Work out the finished part from the listing and answer in its coordinate system (mm). Face numbers are marked on the shaded views. Coordinates: 2 decimals unless noted, no trailing zeros. Loops run counter-clockwise (first coordinate to the right, second up) from the corner with the lowest first, then second, coordinate; pieces in that order, holes last. Notation, with made-up numbers: (88, 4) -> (113, 4) arc R14 cw to (113, 21) -> close; hole circle Ø6 at (66.25, -0.5). An arc over 180 degrees is marked (long way). Answer as CSV lines item,"result".
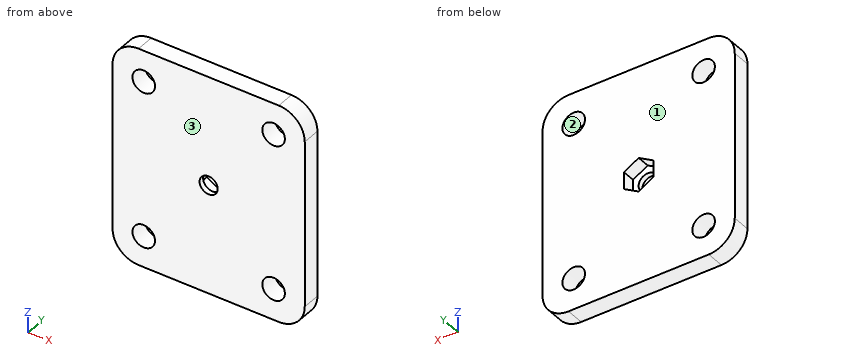
Autodesk Inventor part; units mm, degrees
ref_plane "YZ Plane" through (0, 0, 0) normal (1, 0, 0) x (0, 1, 0)
ref_plane "XZ Plane" through (0, 0, 0) normal (0, 1, 0) x (-1, 0, 0)
ref_plane "XY Plane" through (0, 0, 0) normal (0, 0, 1) x (1, 0, 0)
sketch "Sketch1" plane through (0, 0, 0) normal (0, 1, 0) x (-1, 0, 0)
  line L0 (37, 42) -> (-37, 42)
  line L1 (-37, 42) -> (-37, -42)
  line L2 (-37, -42) -> (37, -42)
  line L3 (37, -42) -> (37, 42)
  line L4 (37, 42) -> (-37, -42) construction
  line L5 (-37, 42) -> (37, -42) construction
  circle A0 centre (25, 30) radius 4.35
  circle A1 centre (25, -30) radius 4.35
  circle A2 centre (-25, 30) radius 4.35
  circle A3 centre (-25, -30) radius 4.35
  point P0 (0, 0)
  dimension "d0" = 74
  dimension "d1" = 84
  dimension "d4" = 60
  dimension "d7" = 50
  dimension "d10" = 8.7
  dimension "d11" = 12
  dimension "d12" = 12
extrude "Extrusion1" add sketch "Sketch1" along normal blind 7
fillet "Fillet1" radius 10 4 edges at (-37, 3.5, 42) (37, 3.5, 42) (37, 3.5, -42) (-37, 3.5, -42)
sketch "Sketch2" plane through (0, 7, 0) normal (0, 1, 0) x (1, 0, 0)
  line L0 (0, 6.5241) -> (5.65, 3.262)
  line L1 (5.65, 3.262) -> (5.65, -3.262)
  line L2 (5.65, -3.262) -> (0, -6.5241)
  line L3 (0, -6.5241) -> (-5.65, -3.262)
  line L4 (-5.65, -3.262) -> (-5.65, 3.262)
  line L5 (-5.65, 3.262) -> (0, 6.5241)
  point P0 (0, 0)
  point P1 (0, 0)
  dimension "d16" = 11.3
extrude "Extrusion2" cut sketch "Sketch2" against normal blind 5
sketch "Sketch3" plane through (0, 2, 0) normal (0, 1, 0) x (1, 0, 0)
  circle A0 centre (0, 0) radius 3.5
  dimension "d19" = 7
extrude "Extrusion3" cut sketch "Sketch3" against normal through all
properties part number "Yagi_fixed_plate"
(1) For a pull along Y with two mould halves and no side action, classify the marked faces 1, 2 and 3 as pulls with the +Y half, pulls with the -Y half, needs draft (parallel to the pull), parting line crosses it, or undercut.
Computed values:
face 1,"pulls with the +Y half"
face 2,"needs draft"
face 3,"pulls with the -Y half"
(2) Flat-ended cylindrical pins translate along their axes: pin 1 Ø5 at (x, z) = (25, 30) entering from -Y; pin 2 Ø3.5 at (x, z) = (2.5, 2.5) entering from +Y. Find the tip coordinate at first contact, or state that the pin passes through.
Computed values:
pin 1,"through"
pin 2,"y = 2"
(3) A cutting plane is placed at D-D, the plane z = -30. Write down the section's boundary in (x, y), and give its area (3 significant figures).
Computed values:
outline,"(-37, 0) -> (-29.35, 0) -> (-29.35, 7) -> (-37, 7) -> close; (-20.65, 0) -> (20.65, 0) -> (20.65, 7) -> (-20.65, 7) -> close; (29.35, 0) -> (37, 0) -> (37, 7) -> (29.35, 7) -> close"
area,"396 mm2"
(4) A cutting plane is placed at B-B, the plane y = 4.25. Write down the section's boundary in (x, z), and give its area (3 significant figures).
Computed values:
outline,"(-37, -32) arc R10 ccw to (-27, -42) -> (27, -42) arc R10 ccw to (37, -32) -> (37, 32) arc R10 ccw to (27, 42) -> (-27, 42) arc R10 ccw to (-37, 32) -> close; hole circle Ø8.7 at (-25, -30); hole circle Ø8.7 at (-25, 30); hole (-5.65, -3.26) -> (0, -6.52) -> (5.65, -3.26) -> (5.65, 3.26) -> (0, 6.52) -> (-5.65, 3.26) -> close; hole circle Ø8.7 at (25, -30); hole circle Ø8.7 at (25, 30)"
area,"5,780 mm2"
(5) A cutting plane is placed at C-C, the plane x = 25. Write down the section's boundary in (y, z), and give its area (3 significant figures).
Computed values:
outline,"(0, -42) -> (7, -42) -> (7, -34.35) -> (0, -34.35) -> close; (0, -25.65) -> (7, -25.65) -> (7, 25.65) -> (0, 25.65) -> close; (0, 34.35) -> (7, 34.35) -> (7, 42) -> (0, 42) -> close"
area,"466 mm2"
(6) A cutting plane is placed at A-A, the plane z = 0. Write down the section's boundary in (x, y), and give its area (4 significant figures).
Computed values:
outline,"(-37, 0) -> (-3.5, 0) -> (-3.5, 2) -> (-5.65, 2) -> (-5.65, 7) -> (-37, 7) -> close; (3.5, 0) -> (37, 0) -> (37, 7) -> (5.65, 7) -> (5.65, 2) -> (3.5, 2) -> close"
area,"447.5 mm2"
(7) Consider line 1 along Z through (x, y) = (25, 2.5); line 2 along Z through (x, y) = (23.5, 1.5); line 3 along Z through (x, y) = (0, 4.75). Determine where each line is inside the solid, lowest interval first.
Computed values:
line 1,"-42 to -34.35, -25.65 to 25.65, 34.35 to 42"
line 2,"-42 to -34.08, -25.92 to 25.92, 34.08 to 42"
line 3,"-42 to -6.52, 6.52 to 42"
